Geometry check sheet. Reference: drawing and pictorial views, mm from the part's lowest x, y, z. A direction names the side the tool comes from. Round coordinates to 2 decimals unless told otherwise and drop trailing zeros. Write each loop counter-clockwise with the first axis right and the second up, starting at its lowest first coordinate (ties: lowest second). Pieces come first, ordered by that corner, then holes. Notation, with made-up numbers: M 75.5,-13 L 132.5,-13 A18 ccw 132.5,11 Z; hole C 11,25 d4. An arc over 180 degrees is marked long. Use a Markdown table: item, result. Add a question column.
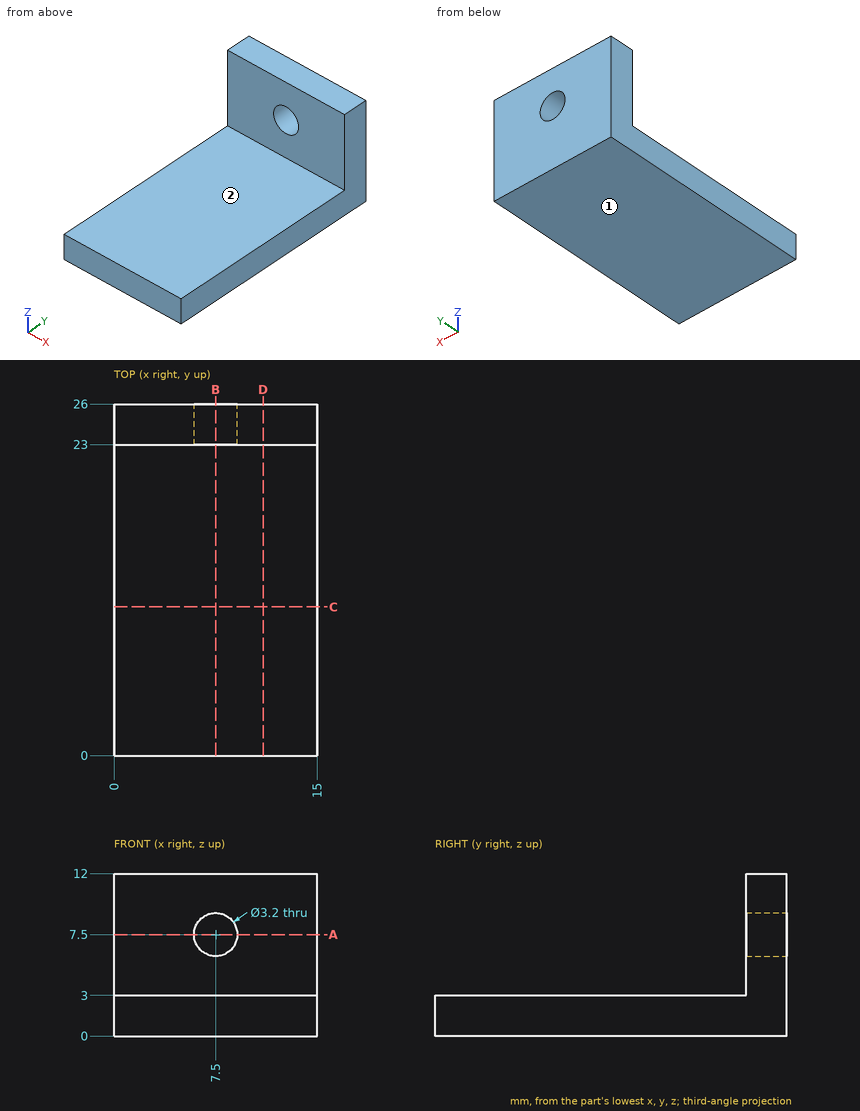
1. Cross-section at B-B on x = 7.5. Enter the section's corners in (y, z).
2. Access from +Z, -Z, +X, -X, +Y, -Y to the whole of each face (thin tool, end or side, straight path). Record for the marked faces 1 and 2.
3. Depth check by flat-ended pin: pin 1 Ø2 at (x, y) = (11.5, 15) entering from +Z. Enter the tip coordinate at first touch or a pass-through.
4. Cross-section at D-D on x = 11. Enter the section's corners in (y, z).
5. Scan lines: line 1 along Z through (x, y) = (7.5, 23.65); line 2 along Z through (x, y) = (8.75, 8.5); line 3 along Y through (x, z) = (13.5, 9.75). Record each from-to range of solid material in increasing order. Write a range as from..to.
6. Cross-section at C-C on y = 11. Enter the section's corners in (x, z), plus the area to 3 significant figures.
7. Cross-section at A-A on z = 7.5. Enter the section's corners in (x, y), plus the area to 3 significant figures.
Answer:
| question | item | result |
|---|---|---|
| 1 | outline | M 0,0 L 26,0 L 26,5.9 L 23,5.9 L 23,3 L 0,3 Z; M 23,9.1 L 26,9.1 L 26,12 L 23,12 Z |
| 2 | face 1 | -Z, +X, -X, +Y, -Y |
| 2 | face 2 | +Z, +X, -X, -Y |
| 3 | pin 1 | stops at z = 3 |
| 4 | outline | M 0,0 L 26,0 L 26,12 L 23,12 L 23,3 L 0,3 Z |
| 5 | line 1 | z = 0..5.9, 9.1..12 |
| 5 | line 2 | z = 0..3 |
| 5 | line 3 | y = 23..26 |
| 6 | outline | M 0,0 L 15,0 L 15,3 L 0,3 Z |
| 6 | area | 45.0 mm^2 |
| 7 | outline | M 0,23 L 5.9,23 L 5.9,26 L 0,26 Z; M 9.1,23 L 15,23 L 15,26 L 9.1,26 Z |
| 7 | area | 35.4 mm^2 |
